Build history of the part. All positions in model axes, mm. A direction names the side the tool comes from. Round coordinates to 2 decimals unless told otherwise and drop trailing zeros. One line per item, written item: value. Start each with the question number.
Item 1: Two-plate mould, pull along X, no slides. Class faces 1 (the flat face through (25, -34, 15.76)), 2 (the flat face through (-16.4, 72.1, 0)): +X half, -X half, draft (parallel to the pull), parting line (faces both ways), or undercut.
Item 2: Tool access for faces 3 (the cylindrical face through (29.137, -27.343, 16.389)), 4 (the flat face through (37, -50.238, 9)), 5 (the flat face through (-159.38, -35.75, 8.46)), 6 (the cylindrical face through (-10.84, 46.15, 13.57)): list every direction of +Z, -Z, +X, -X, +Y, -Y with a clear straight run to the whole face (end or side of a thin tool).
Item 3: Pin check, flat tips, straight feed: pin 1 (9.5 mm diameter, centred on x = -57.22, y = 108.48, fed in from -Z); pin 2 (4.5 mm diameter, centred on x = -57, y = 131.5, fed in from -Z); pin 3 (2.5 mm diameter, centred on x = -51, z = 9, fed in from -Y). Stop position of each tip, or through.
Item 4: Probe L1, parallel to Y at x = -103, z = 7.5; L2, parallel to Y at x = -128, z = 8.5; L3, parallel to X at y = 109, z = 8.5. List the from-to ranges inside material, lowest first.
```python
from build123d import *

# Parameters (mm, degrees)
BOSS_EXTRU_1_DEPTH      = 15
BOSS_EXTRU_2_DEPTH      = 2
ESQUISSE3_W             = 164.930853143
ESQUISSE3_H             = 1.4
BOSS_EXTRU_3_DEPTH      = 11
ENL_V_MAT_EXTRU_1_DEPTH = 2.1
ENL_V_MAT_EXTRU_2_REACH = 232.446
CONG_1_R                = 5
ESQUISSE6_R             = 7.75
ENL_V_MAT_EXTRU_3_DEPTH = 1.24
ESQUISSE7_R             = 2.75
ENL_V_MAT_EXTRU_4_DEPTH = 1.14
CONG_2_R                = 5
ENL_V_MAT_EXTRU_6_DEPTH = 2
ESQUISSE8_R             = 2.75
ENL_V_MAT_EXTRU_5_DEPTH = 4


with BuildPart() as part:
    # Esquisse1 → Boss.-Extru.1 (new body)
    with BuildSketch(Plane.XY):
        Polygon((-169.71822613, -51.377911564), (-57.21822613, 143.477804287), (55.28177387, -51.377911564), align=None)
        Polygon((46.621519833, -46.377911564), (-161.057972092, -46.377911564), (-57.21822613, 133.477804287), align=None, mode=Mode.SUBTRACT)
    extrude(amount=BOSS_EXTRU_1_DEPTH)

    # Esquisse2 → Boss.-Extru.2 (add)
    with BuildSketch(Plane.XY.offset(15)):
        Polygon((-57.21822613, 143.477804287), (-169.71822613, -51.377911564), (55.28177387, -51.377911564), align=None)
    extrude(amount=BOSS_EXTRU_2_DEPTH)

    # Esquisse3 → Boss.-Extru.3 (add)
    with BuildSketch(Plane(origin=(0, 0, 15), x_dir=(-1, 0, 0), z_dir=(0, 0, -1))):
        Polygon((53.949011072, 117.815357706), (-28.5164155, -25.018950984), (-27.303979934, -25.718950984), (55.161446637, 117.115357706), align=None)
        Polygon((149.019751584, -35.527102012), (147.807316018, -36.227102012), (65.341889447, 106.607206677), (66.554325012, 107.307206677), align=None)
        with Locations((51.042590893, -40.677911564)):
            Rectangle(ESQUISSE3_W, ESQUISSE3_H)
    extrude(amount=BOSS_EXTRU_3_DEPTH)

    # Esquisse4 → Enlèv. mat.-Extru.1 (cut)
    with BuildSketch(Plane(origin=(19.214042099, 11.093232378, 0), x_dir=(0, 0, -1), z_dir=(0.8660254037844387, 0.5000000000000001, 0))):
        with BuildLine():
            Line((-12.65, 52.464536457), (-12.65, 28.264536457))
            ThreePointArc((-12.65, 28.264536457), (-8.5, 24.114536457), (-4.35, 28.264536457))
            Line((-4.35, 28.264536457), (-4.35, 52.464536457))
            ThreePointArc((-4.35, 52.464536457), (-8.5, 56.614536457), (-12.65, 52.464536457))
        make_face()
    enl_v_mat_extru_1 = extrude(amount=-ENL_V_MAT_EXTRU_1_DEPTH, mode=Mode.SUBTRACT)

    # Esquisse5 → Enlèv. mat.-Extru.2 (cut, up to next)
    with BuildSketch(Plane(origin=(17.395388751, 10.043232378, 0), x_dir=(0, 0, -1), z_dir=(0.8660254037844386, 0.5000000000000003, 0)), mode=Mode.PRIVATE) as enl_v_mat_extru_2_sk1:
        with BuildLine():
            Line((-11.65, 52.464536457), (-11.65, 28.264536457))
            ThreePointArc((-11.65, 28.264536457), (-8.5, 25.114536457), (-5.35, 28.264536457))
            Line((-5.35, 28.264536457), (-5.35, 52.464536457))
            ThreePointArc((-5.35, 52.464536457), (-8.5, 55.614536457), (-11.65, 52.464536457))
        make_face()
    enl_v_mat_extru_2_tool1 = extrude(enl_v_mat_extru_2_sk1.sketch, amount=-ENL_V_MAT_EXTRU_2_REACH, mode=Mode.PRIVATE) & part.part
    enl_v_mat_extru_2 = enl_v_mat_extru_2_tool1.solids().sort_by_distance((-2.786879, 44.999946, 8.5))[0]
    add(enl_v_mat_extru_2, mode=Mode.SUBTRACT)

    # Congé1
    cong_1_edges = [part.edges().sort_by_distance(p)[0] for p in [
        (46.621519833, -46.377911564, 7.5),
        (-57.21822613, 133.477804287, 7.5),
        (-161.057972092, -46.377911564, 7.5),
        (-169.71822613, -51.377911564, 8.5),
        (-57.21822613, 143.477804287, 8.5),
        (55.28177387, -51.377911564, 8.5),
    ]]
    fillet(cong_1_edges, radius=CONG_1_R)

    # Symétrie1: Enlèv. mat.-Extru.1, Enlèv. mat.-Extru.2 across plane
    add(enl_v_mat_extru_1.mirror(Plane(origin=(-8.426844836, -14.595723404, 0), x_dir=(0, 0, 1), z_dir=(0.5000000000000001, 0.8660254037844386, 0))), mode=Mode.SUBTRACT)
    add(enl_v_mat_extru_2.mirror(Plane(origin=(-8.426844836, -14.595723404, 0), x_dir=(0, 0, 1), z_dir=(0.5000000000000001, 0.8660254037844386, 0))), mode=Mode.SUBTRACT)

    # Esquisse6 → Enlèv. mat.-Extru.3 (cut)
    with BuildSketch(Plane.XY.offset(17)):
        with Locations((-57.21822613, 108.477804287)):
            Circle(ESQUISSE6_R)
        with Locations(Location((-139.407336997, -33.877911564, 0), (0, 0, 180))):
            Circle(ESQUISSE6_R)
        with Locations((24.970884738, -33.877911564)):
            Circle(ESQUISSE6_R)
    extrude(amount=-ENL_V_MAT_EXTRU_3_DEPTH, mode=Mode.SUBTRACT)

    # Esquisse7 → Enlèv. mat.-Extru.4 (cut)
    with BuildSketch(Plane.XZ.offset(51.377911564)):
        with Locations((36.621519833, 8.5)):
            Circle(ESQUISSE7_R)
        with Locations(Location((-151.057972092, 8.5, 0), (0, 0, 180))):
            Circle(ESQUISSE7_R)
    enl_v_mat_extru_4 = extrude(amount=-ENL_V_MAT_EXTRU_4_DEPTH, mode=Mode.SUBTRACT)

    # Symétrie2: Enlèv. mat.-Extru.4 across plane
    add(enl_v_mat_extru_4.mirror(Plane(origin=(-8.426844836, -14.595723404, 0), x_dir=(0, 0, 1), z_dir=(0.5000000000000001, 0.8660254037844386, 0))), mode=Mode.SUBTRACT)

    # Symétrie3: Enlèv. mat.-Extru.4 across plane
    add(enl_v_mat_extru_4.mirror(Plane(origin=(-20.182268228, 34.956713983, 0), x_dir=(0, 0, 1), z_dir=(0.5000000000000001, -0.8660254037844387, 0))), mode=Mode.SUBTRACT)

    # Congé2
    cong_2_edges = [part.edges().sort_by_distance(p)[0] for p in [
        (-12.716297786, 46.398203361, 15),
        (-107.787038298, 35.890052333, 15),
        (-51.042590892, -41.377911564, 15),
    ]]
    fillet(cong_2_edges, radius=CONG_2_R - 0.0001)  # a hair under: the kernel refuses the full size

    # Esquisse9 → Enlèv. mat.-Extru.6 (cut)
    with BuildSketch(Plane(origin=(0, 0, 0), x_dir=(-1, 0, 0), z_dir=(0, 0, -1))):
        with BuildLine():
            Line((164.089061005, -44.627911564), (60.249315043, 135.227804287))
            ThreePointArc((60.249315043, 135.227804287), (57.21822613, 136.977804287), (54.187137216, 135.227804287))
            Line((54.187137216, 135.227804287), (-49.652608746, -44.627911564))
            ThreePointArc((-49.652608746, -44.627911564), (-49.652608746, -48.127911564), (-46.621519833, -49.877911564))
            Line((-46.621519833, -49.877911564), (161.057972092, -49.877911564))
            ThreePointArc((161.057972092, -49.877911564), (164.089061005, -48.127911564), (164.089061005, -44.627911564))
        make_face()
    extrude(amount=-ENL_V_MAT_EXTRU_6_DEPTH, mode=Mode.SUBTRACT)

    # Esquisse8 → Enlèv. mat.-Extru.5 (cut)
    with BuildSketch(Plane(origin=(0, 0, 0), x_dir=(-1, 0, 0), z_dir=(0, 0, -1))):
        with Locations((-45.914902423, -45.969945813)):
            Circle(ESQUISSE8_R)
        with Locations((57.21822613, 132.661872783)):
            Circle(ESQUISSE8_R)
        with Locations((160.351354682, -45.969945813)):
            Circle(ESQUISSE8_R)
    extrude(amount=-ENL_V_MAT_EXTRU_5_DEPTH, mode=Mode.SUBTRACT)


solid = part.part
```
Output:
1. face 1: undercut
1. face 2: draft
2. face 3: +Z
2. face 4: -Y
2. face 5: none
2. face 6: -Z
3. pin 1: stops at z = 15
3. pin 2: stops at z = 2
3. pin 3: stops at y = -41.38
4. L1: y = -51.38 to -46.38, -41.38 to -39.98, 41.38 to 44.18, 54.18 to 64.18
4. L2: y = -51.38 to -46.38, -41.38 to -39.98, -1.92 to 0.88, 10.88 to 20.88
4. L3: x = -77.12 to -71.35, -50.48 to -48.86, -43.09 to -37.31
